Can you work these out from the model? Positions are in its coordinate system, mm. Round coordinates to 2 decimals unless told otherwise and drop trailing zeros. Order: outer loops, then holes, each group sorted by start corner. A loop starts at its lowest first (then second) coordinate and runs counter-clockwise, first axis right, second up. Notation, with made-up numbers: (-35, 44) -> (-26, 44) arc R19 ccw to (-26, 64) -> close; hole circle Ø6 at (64.5, -2.5). An arc over 180 degrees is marked (long way). Use a Markdown table: item, result. Add a question column.
Q1. If we section it at D-D on z = 25: List the corners of the cut face in (x, y) for me.
Q2. If we section it at B-B on x = 0: List the corners of the cut face in (y, z) for me, plus the area to 4 significant figures.
Q3. If we section it at A-A on z = -29: List the corners of the cut face in (x, y) for me.
Q4. I need wall thicknesses on line 1 along Z through (x, y) = (0, 0.05); line 2 along Z through (x, y) = (4.5, -0.7); line 3 along X through (y, z) = (-1.5, -23). Which ranges of each line are inside material? Lowest first, please. Write a range as [from, to].
Q5. If we section it at C-C on y = -0.15: List the corners of the cut face in (x, z) for me, plus the area to 3 significant figures.
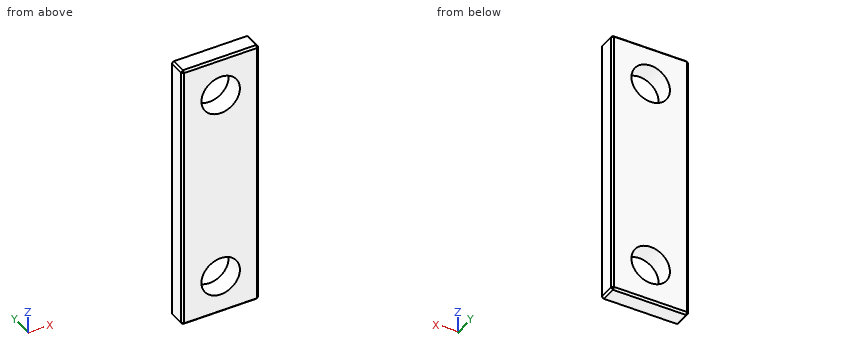
Autodesk Inventor part; units mm, degrees
ref_plane "YZ Plane" through (0, 0, 0) normal (1, 0, 0) x (0, 1, 0)
ref_plane "XZ Plane" through (0, 0, 0) normal (0, 1, 0) x (-1, 0, 0)
ref_plane "XY Plane" through (0, 0, 0) normal (0, 0, 1) x (1, 0, 0)
sketch "Sketch1" plane through (0, 0, 0) normal (0, 1, 0) x (-1, 0, 0)
  circle A0 centre (0, 25) radius 5
  circle A1 centre (0, -25) radius 5
  line L0 (10, 35) -> (10, -35)
  line L1 (-10, -35) -> (-10, 35)
  line L2 (10, -35) -> (-10, -35)
  line L3 (10, 35) -> (-10, 35)
  line L4 (0, -25) -> (0, 25) construction
  point P0 (0, 0)
  point P1 (10, 0)
  point P2 (0, -35)
  point P3 (0, 35)
  point P4 (0, 0)
  dimension "d1" = 10
  dimension "d5" = 20
  dimension "d6" = 10
  dimension "d7" = 50
extrude "Extrusion1" add sketch "Sketch1" along normal mid plane 5
chamfer "Chamfer2" distance 0.5 angle 45 12 edges at (10, 2.5, 0) (0, 2.5, 35) (-10, 2.5, 0) (0, 2.5, -35) (0, -2.5, 35) (10, -2.5, 0) (-10, -2.5, 0) (0, -2.5, -35) (10, 0, 35) (-10, 0, 35) (10, 0, -35) (-10, 0, -35)
equation "\"d6\" = d5 - d1"
properties part number "link_c" material "Aluminium 6082 T6"
Answer below:
| question | item | result |
|---|---|---|
| 1 | outline | (-10, -2) -> (-9.5, -2.5) -> (-5, -2.5) -> (-5, 2.5) -> (-9.5, 2.5) -> (-10, 2) -> close; (5, -2.5) -> (9.5, -2.5) -> (10, -2) -> (10, 2) -> (9.5, 2.5) -> (5, 2.5) -> close |
| 2 | outline | (-2.5, -34.5) -> (-2, -35) -> (2, -35) -> (2.5, -34.5) -> (2.5, -30) -> (-2.5, -30) -> close; (-2.5, -20) -> (2.5, -20) -> (2.5, 20) -> (-2.5, 20) -> close; (-2.5, 30) -> (2.5, 30) -> (2.5, 34.5) -> (2, 35) -> (-2, 35) -> (-2.5, 34.5) -> close |
| 2 | area | 249.5 mm² |
| 3 | outline | (-10, -2) -> (-9.5, -2.5) -> (-3, -2.5) -> (-3, 2.5) -> (-9.5, 2.5) -> (-10, 2) -> close; (3, -2.5) -> (9.5, -2.5) -> (10, -2) -> (10, 2) -> (9.5, 2.5) -> (3, 2.5) -> close |
| 4 | line 1 | [-35, -30], [-20, 20], [30, 35] |
| 4 | line 2 | [-35, -27.18], [-22.82, 22.82], [27.18, 35] |
| 4 | line 3 | [-10, -4.58], [4.58, 10] |
| 5 | outline | (-10, -34.5) -> (-9.5, -35) -> (9.5, -35) -> (10, -34.5) -> (10, 34.5) -> (9.5, 35) -> (-9.5, 35) -> (-10, 34.5) -> close; hole circle Ø10 at (0, -25); hole circle Ø10 at (0, 25) |
| 5 | area | 1,240 mm² |
